from build123d import *

# Parameters (mm, degrees)
BOSS_EXTRUDE1_DEPTH = 2
FILLET2_R           = 1
SKETCH2_W           = 12
SKETCH2_H           = 22
CUT_EXTRUDE1_DEPTH  = 10
FILLET3_R           = 1


with BuildPart() as part:
    # Sketch1 → Boss-Extrude1 (new body)
    with BuildSketch(Plane.XY):
        with BuildLine():
            Line((0, 0), (23, 0))
            Line((23, 0), (23, 34.769696007))
            ThreePointArc((23, 34.769696007), (22.258788496, 34.942088629), (21.5, 35))
            Line((21.5, 35), (1.5, 35))
            ThreePointArc((1.5, 35), (0.741211504, 34.942088629), (0, 34.769696007))
            Line((0, 34.769696007), (0, 0))
        make_face()
    extrude(amount=BOSS_EXTRUDE1_DEPTH)

    # Fillet2
    fillet2_edges = [part.edges().sort_by_distance(p)[0] for p in [
        (0, 34.769696007, 1),
        (23, 34.769696007, 1),
        (23, 0, 1),
        (0, 0, 1),
    ]]
    fillet(fillet2_edges, radius=FILLET2_R)

    # Sketch2 → Cut-Extrude1 (cut)
    with BuildSketch(Plane.XY.offset(2)):
        with Locations((11.5, 11)):
            Rectangle(SKETCH2_W, SKETCH2_H)
    extrude(amount=-CUT_EXTRUDE1_DEPTH, mode=Mode.SUBTRACT)

    # Fillet3
    fillet3_edges = [part.edges().sort_by_distance(p)[0] for p in [
        (5.5, 0, 1),
        (5.5, 22, 1),
        (17.5, 22, 1),
        (17.5, 0, 1),
    ]]
    fillet(fillet3_edges, radius=FILLET3_R)


solid = part.part
Geometry: final body of the model. Coordinates: model frame, mm. A direction names the side the tool comes from. Coordinates: 2 decimals unless noted, no trailing zeros. Loops run counter-clockwise (first coordinate to the right, second up) from the corner with the lowest first, then second, coordinate; pieces in that order, holes last. Notation, with made-up numbers: M 8.5,51 L 18.5,51 A14 ccw 18.5,55 Z; hole C 71,13 d1. An arc over 180 degrees is marked long. One line per item, written item: value. Start each with the question number.
1) Cut plane C-C (x = 11.25). Return loops of the section in (y, z).
2) Cut plane B-B (z = 0.7). Return loops of the section in (x, y) (3 decimals), then the cut area to 3 significant figures.
3) Reachability of faces 1 (the cylindrical face through (0.26, 34.64, 1.01)), 2 (the flat face through (5.5, 11, 1)) from +Z, -Z, +X, -X, +Y, -Y: full face, straight path, thin tool, end or side. Return the list, or none.
4) Material intervals for L1, parallel to X at y = 8, z = 1.95; L2, parallel to Y at x = 8.5, z = 1.3; L3, parallel to Y at x = 4.75, z = 1.65, sorted ascending. Write a range as from..to.
5) Cut plane A-A (y = 16). Return loops of the section in (x, z), then the cut area to 3 significant figures.
6) Pin query (flat end, axial travel): P1, Ø1.5, axis at x = 16.5, y = 21.5, coming from the +Z side. Return the tip coordinate at first contact, or that it passes through.
Evaluation:
1. outline: M 22,0 L 35,0 L 35,2 L 22,2 Z
2. outline: M 0,1 A1 ccw 1,0 L 4.5,0 A1 ccw 5.5,1 L 5.5,21 A1 cw 6.5,22 L 16.5,22 A1 cw 17.5,21 L 17.5,1 A1 ccw 18.5,0 L 22,0 A1 ccw 23,1 L 23,33.969 A1 ccw 22.125,34.961 A5 ccw 21.5,35 L 1.5,35 A5 ccw 0.875,34.961 A1 ccw 0,33.969 Z
2. area: 540 mm^2
3. face 1: +Z, -Z, -X, +Y
3. face 2: +Z, -Z, -Y
4. L1: 0..5.5, 17.5..23
4. L2: 22..35
4. L3: 0.03..35
5. outline: M 0,0 L 5.5,0 L 5.5,2 L 0,2 Z; M 17.5,0 L 23,0 L 23,2 L 17.5,2 Z
5. area: 22.0 mm^2
6. P1: z = 2
